Geometry check sheet. Reference: the model listing, model coordinates, mm. Face numbers are marked on the shaded views. A direction names the side the tool comes from. Coordinates: 2 decimals unless noted, no trailing zeros. Write each loop counter-clockwise with the first axis right and the second up, starting at its lowest first coordinate (ties: lowest second). Pieces come first, ordered by that corner, then holes. Notation, with made-up numbers: (-23.75, 41.25) -> (31.25, 41.25) arc R20 ccw to (31.25, 65.25) -> close; hole circle Ø7 at (9.5, 6). An arc over 180 degrees is marked (long way). Answer in a Markdown table with one row per item. Add a question column.
1. Scan lines: L1, parallel to Y at x = -0.5, z = 1; L2, parallel to Z at x = 3.5, y = 6.5; L3, parallel to Y at x = 3, z = 2. Record each from-to range of solid material in increasing order. Write a range as from..to.
2. Depth check by flat-ended pin: P1, Ø0.6, axis at y = 7.5, z = 1.5, coming from the -X side (3 decimals); P2, Ø2, axis at x = 0.5, y = 2.5, coming from the -Z side. Enter the tip coordinate at first touch or a pass-through.
3. Set-up check for the marked faces 5, 6 and 7: record each of +Z, -Z, +X, -X, +Y, -Y from which the full face is reachable in a straight line by a thin tool's end or side.
4. Mould release check, pull along Y, two halves, no side actions. Record for the marked faces 1, 2, 3 and 4: pulls with the +Y half, pulls with the -Y half, needs draft (parallel to the pull), parting line crosses it, or undercut.
5. Cross-section at C-C on x = 4. Record the cut outline in (y, z), and give its area (3 significant figures).
6. Cross-section at D-D on z = 0.5. Record the cut outline in (x, y) (3 decimals), and give its area (3 significant figures).
7. Cross-section at B-B on y = 5.75. Record the cut outline in (x, z) (3 decimals), and give its area (3 significant figures).
8. Cross-section at A-A on z = -0.75. Record the cut outline in (x, y).
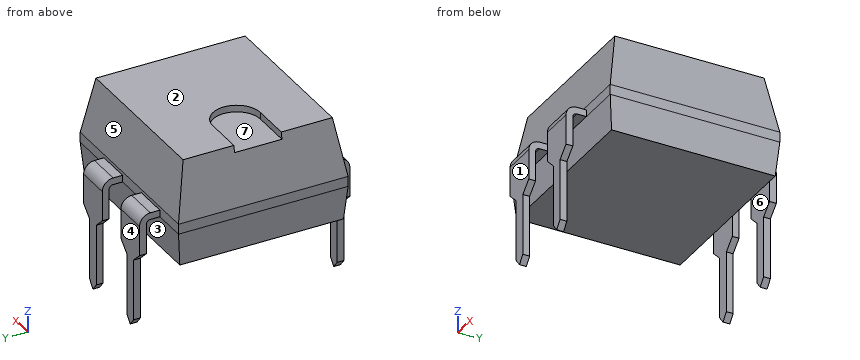
```python
from build123d import *
from OCP.BRepFilletAPI import BRepFilletAPI_MakeChamfer

# Parameters (mm, degrees)
SKETCH1_W                = 6.705
SKETCH1_H                = 6.35
BASE_EXTRUDE_DEPTH       = 3.81
CHAMFER1_SIZE            = 2.159
CHAMFER1_SIZE2           = 0.380689951
CHAMFER2_SIZE            = 1.27
CHAMFER2_SIZE2           = 0.111110603
CUT_EXTRUDE1_START       = 3.937
CUT_EXTRUDE1_DEPTH       = 0.254
BOSS_EXTRUDE_THIN3_DEPTH = 0.635
CUT_EXTRUDE3_DEPTH       = 10.549085035
CUT_EXTRUDE4_DEPTH       = 10.549085035
LPATTERN2_COUNT          = 2
LPATTERN2_PITCH          = 2.54
MIRROR1_COPY_1_DEPTH     = 0.635
MIRROR1_COPY_2_DEPTH     = 10.549085035
MIRROR1_COPY_3_DEPTH     = 10.549085035


# Read off the part's stored shape, not the designer's step: Cut-Extrude1
with BuildPart() as part:
    # Sketch1 → Base-Extrude (new body)
    with BuildSketch(Plane.XY.offset(0.381)):
        with Locations((1.4475, 3.937)):
            Rectangle(SKETCH1_W, SKETCH1_H)
    extrude(amount=BASE_EXTRUDE_DEPTH)

    # Chamfer1: one chamfer whose edges measure the first distance from different faces: ONE call of the kernel's chamfer builder (chamfer() names one face for all edges)
    chamfer1_edges_1 = [part.edges().sort_by_distance(p)[0] for p in [
        (4.8, 3.937, 4.191),
    ]]
    chamfer1_side_1 = [part.faces().sort_by_distance(p)[0] for p in [
        (4.8, 3.937, 2.286),
    ]]
    chamfer1_edges_2 = [part.edges().sort_by_distance(p)[0] for p in [
        (1.4475, 7.112, 4.191),
    ]]
    chamfer1_side_2 = [part.faces().sort_by_distance(p)[0] for p in [
        (1.4475, 7.112, 2.286),
    ]]
    chamfer1_edges_3 = [part.edges().sort_by_distance(p)[0] for p in [
        (-1.905, 3.937, 4.191),
    ]]
    chamfer1_side_3 = [part.faces().sort_by_distance(p)[0] for p in [
        (-1.905, 3.937, 2.286),
    ]]
    chamfer1_edges_4 = [part.edges().sort_by_distance(p)[0] for p in [
        (1.4475, 0.762, 4.191),
    ]]
    chamfer1_side_4 = [part.faces().sort_by_distance(p)[0] for p in [
        (1.4475, 0.762, 2.286),
    ]]
    chamfer1 = BRepFilletAPI_MakeChamfer(part.part.solid().wrapped)
    for e in chamfer1_edges_1:
        chamfer1.Add(CHAMFER1_SIZE, CHAMFER1_SIZE2, e.wrapped, chamfer1_side_1[0].wrapped)  # the first distance lies on this face
    for e in chamfer1_edges_2:
        chamfer1.Add(CHAMFER1_SIZE, CHAMFER1_SIZE2, e.wrapped, chamfer1_side_2[0].wrapped)  # the first distance lies on this face
    for e in chamfer1_edges_3:
        chamfer1.Add(CHAMFER1_SIZE, CHAMFER1_SIZE2, e.wrapped, chamfer1_side_3[0].wrapped)  # the first distance lies on this face
    for e in chamfer1_edges_4:
        chamfer1.Add(CHAMFER1_SIZE, CHAMFER1_SIZE2, e.wrapped, chamfer1_side_4[0].wrapped)  # the first distance lies on this face
    add(Compound.cast(chamfer1.Shape()), mode=Mode.REPLACE)

    # Chamfer2: one chamfer whose edges measure the first distance from different faces: ONE call of the kernel's chamfer builder (chamfer() names one face for all edges)
    chamfer2_edges_1 = [part.edges().sort_by_distance(p)[0] for p in [
        (1.4475, 7.112, 0.381),
    ]]
    chamfer2_side_1 = [part.faces().sort_by_distance(p)[0] for p in [
        (1.4475, 7.112, 1.2065),
    ]]
    chamfer2_edges_2 = [part.edges().sort_by_distance(p)[0] for p in [
        (4.8, 3.937, 0.381),
    ]]
    chamfer2_side_2 = [part.faces().sort_by_distance(p)[0] for p in [
        (4.8, 3.937, 1.2065),
    ]]
    chamfer2_edges_3 = [part.edges().sort_by_distance(p)[0] for p in [
        (1.4475, 0.762, 0.381),
    ]]
    chamfer2_side_3 = [part.faces().sort_by_distance(p)[0] for p in [
        (1.4475, 0.762, 1.2065),
    ]]
    chamfer2_edges_4 = [part.edges().sort_by_distance(p)[0] for p in [
        (-1.905, 3.937, 0.381),
    ]]
    chamfer2_side_4 = [part.faces().sort_by_distance(p)[0] for p in [
        (-1.905, 3.937, 1.2065),
    ]]
    chamfer2 = BRepFilletAPI_MakeChamfer(part.part.solid().wrapped)
    for e in chamfer2_edges_1:
        chamfer2.Add(CHAMFER2_SIZE, CHAMFER2_SIZE2, e.wrapped, chamfer2_side_1[0].wrapped)  # the first distance lies on this face
    for e in chamfer2_edges_2:
        chamfer2.Add(CHAMFER2_SIZE, CHAMFER2_SIZE2, e.wrapped, chamfer2_side_2[0].wrapped)  # the first distance lies on this face
    for e in chamfer2_edges_3:
        chamfer2.Add(CHAMFER2_SIZE, CHAMFER2_SIZE2, e.wrapped, chamfer2_side_3[0].wrapped)  # the first distance lies on this face
    for e in chamfer2_edges_4:
        chamfer2.Add(CHAMFER2_SIZE, CHAMFER2_SIZE2, e.wrapped, chamfer2_side_4[0].wrapped)  # the first distance lies on this face
    add(Compound.cast(chamfer2.Shape()), mode=Mode.REPLACE)

    # Cut-Extrude1 outline → Cut-Extrude1 (cut)
    with BuildSketch(Plane.XY.offset(CUT_EXTRUDE1_START)):
        with BuildLine():
            Line((-0.099439262, 4.829907029), (-3, 4.829907029))
            Line((-3, 4.829907029), (-3, 3.054205915))
            Line((-3, 3.054205915), (-0.099439262, 3.054205915))
            ThreePointArc((-0.099439262, 3.054205915), (0.788411294, 3.942056472), (-0.099439262, 4.829907029))
        make_face()
    extrude(amount=CUT_EXTRUDE1_DEPTH, mode=Mode.SUBTRACT)

    # Sketch4 → Boss-Extrude-Thin3 (add, symmetric)
    with BuildSketch(Plane(origin=(0, 0, 0), x_dir=(0, 0, -1), z_dir=(1, 0, 0))):
        with BuildLine():
            Line((2.5654, 0), (-1.4986, 0))
            ThreePointArc((-1.4986, 0), (-1.785968196, 0.119031804), (-1.905, 0.4064))
            Line((-1.905, 0.4064), (-1.905, 1.120296425))
            Line((-1.905, 1.120296425), (-1.651, 1.120296425))
            Line((-1.651, 1.120296425), (-1.651, 0.4064))
            ThreePointArc((-1.651, 0.4064), (-1.606363073, 0.298636927), (-1.4986, 0.254))
            Line((-1.4986, 0.254), (2.5654, 0.254))
            Line((2.5654, 0.254), (2.5654, 0))
        make_face()
    boss_extrude_thin3 = extrude(amount=BOSS_EXTRUDE_THIN3_DEPTH, both=True)

    # Sketch8 → Cut-Extrude3 (cut, through all)
    with BuildSketch(Plane.XZ):
        Polygon((-0.635, 0.381), (-0.2286, 0), (-0.2286, -2.286), (0, -2.5654), (-0.635, -2.5654), align=None)
    cut_extrude3 = extrude(amount=-CUT_EXTRUDE3_DEPTH, mode=Mode.SUBTRACT)

    # Sketch9 → Cut-Extrude4 (cut, through all)
    with BuildSketch(Plane.XZ):
        Polygon((0.635, 0.381), (0.2286, 0), (0.2286, -2.286), (0, -2.5654), (0.635, -2.5654), align=None)
    cut_extrude4 = extrude(amount=-CUT_EXTRUDE4_DEPTH, mode=Mode.SUBTRACT)

    # LPattern2: Boss-Extrude-Thin3, Cut-Extrude3, Cut-Extrude4 ×2
    with Locations(*[(i * LPATTERN2_PITCH, 0, 0) for i in range(1, LPATTERN2_COUNT)]):
        add(boss_extrude_thin3)
        add(cut_extrude3, mode=Mode.SUBTRACT)
        add(cut_extrude4, mode=Mode.SUBTRACT)

    # Mirror1: Boss-Extrude-Thin3, Cut-Extrude3, Cut-Extrude4 across plane
    add(boss_extrude_thin3.mirror(Plane.ZX.offset(3.937)))
    add(cut_extrude3.mirror(Plane.ZX.offset(3.937)), mode=Mode.SUBTRACT)
    add(cut_extrude4.mirror(Plane.ZX.offset(3.937)), mode=Mode.SUBTRACT)

    # Mirror1 copy 1 sketch → Mirror1 copy 1 (add, symmetric)
    with BuildSketch(Plane(origin=(2.54, 7.874, 0), x_dir=(0, 0, -1), z_dir=(1, 0, 0))):
        with BuildLine():
            Line((2.5654, 0), (-1.4986, 0))
            ThreePointArc((-1.4986, 0), (-1.785968196, -0.119031804), (-1.905, -0.4064))
            Line((-1.905, -0.4064), (-1.905, -1.120296425))
            Line((-1.905, -1.120296425), (-1.651, -1.120296425))
            Line((-1.651, -1.120296425), (-1.651, -0.4064))
            ThreePointArc((-1.651, -0.4064), (-1.606363073, -0.298636927), (-1.4986, -0.254))
            Line((-1.4986, -0.254), (2.5654, -0.254))
            Line((2.5654, -0.254), (2.5654, 0))
        make_face()
    extrude(amount=MIRROR1_COPY_1_DEPTH, both=True)

    # Mirror1 copy 2 sketch → Mirror1 copy 2 (cut, through all)
    with BuildSketch(Plane(origin=(2.54, 7.874, 0), x_dir=(1, 0, 0), z_dir=(0, 1, 0))):
        Polygon((-0.635, -0.381), (-0.2286, 0), (-0.2286, 2.286), (0, 2.5654), (-0.635, 2.5654), align=None)
    extrude(amount=-MIRROR1_COPY_2_DEPTH, mode=Mode.SUBTRACT)

    # Mirror1 copy 3 sketch → Mirror1 copy 3 (cut, through all)
    with BuildSketch(Plane(origin=(2.54, 7.874, 0), x_dir=(1, 0, 0), z_dir=(0, 1, 0))):
        Polygon((0.635, -0.381), (0.2286, 0), (0.2286, 2.286), (0, 2.5654), (0.635, 2.5654), align=None)
    extrude(amount=-MIRROR1_COPY_3_DEPTH, mode=Mode.SUBTRACT)


solid = part.part
```
Results found:
| question | item | result |
|---|---|---|
| 1 | L1 | y = 0..0.25, 0.82..7.06, 7.62..7.87 |
| 1 | L2 | z = 0.38..4.19 |
| 1 | L3 | y = 0.76..7.11 |
| 2 | P1 | stops at x = -0.635 |
| 2 | P2 | stops at z = 0.38 |
| 3 | face 5 | +Z, +X, -X, +Y |
| 3 | face 6 | -Z, +X, -X |
| 3 | face 7 | +Z, -X |
| 4 | face 1 | pulls with the -Y half |
| 4 | face 2 | needs draft |
| 4 | face 3 | undercut |
| 4 | face 4 | pulls with the +Y half |
| 5 | outline | (0.76, 1.65) -> (0.87, 0.38) -> (7, 0.38) -> (7.11, 1.65) -> (7.11, 2.03) -> (6.73, 4.19) -> (1.14, 4.19) -> (0.76, 2.03) -> close |
| 5 | area | 23.2 mm^2 |
| 6 | outline | (-1.804, 0.863) -> (4.699, 0.863) -> (4.699, 7.011) -> (-1.804, 7.011) -> close; (-0.635, 0) -> (0.635, 0) -> (0.635, 0.254) -> (-0.635, 0.254) -> close; (-0.635, 7.62) -> (0.635, 7.62) -> (0.635, 7.874) -> (-0.635, 7.874) -> close; (1.905, 0) -> (3.175, 0) -> (3.175, 0.254) -> (1.905, 0.254) -> close; (1.905, 7.62) -> (3.175, 7.62) -> (3.175, 7.874) -> (1.905, 7.874) -> close |
| 6 | area | 41.3 mm^2 |
| 7 | outline | (-1.905, 1.651) -> (-1.794, 0.381) -> (4.689, 0.381) -> (4.8, 1.651) -> (4.8, 2.032) -> (4.419, 4.191) -> (-1.524, 4.191) -> (-1.905, 2.032) -> close |
| 7 | area | 24.6 mm^2 |
| 8 | outline | (-0.23, 0) -> (0.23, 0) -> (0.23, 0.25) -> (-0.23, 0.25) -> close; (-0.23, 7.62) -> (0.23, 7.62) -> (0.23, 7.87) -> (-0.23, 7.87) -> close; (2.31, 0) -> (2.77, 0) -> (2.77, 0.25) -> (2.31, 0.25) -> close; (2.31, 7.62) -> (2.77, 7.62) -> (2.77, 7.87) -> (2.31, 7.87) -> close |
